Geometry: final body of the model. Coordinates: model frame, mm. A direction names the side the tool comes from. Give positions to 0.01 mm unless a question says otherwise; leave off trailing zeros. Order: outer loops, then holes, each group sorted by start corner. A loop starts at its lowest first (then second) coordinate and runs counter-clockwise, first axis right, second up. Notation, with made-up numbers: (35.25, -31) -> (81.25, -31) arc R14 cw to (81.25, -26) -> close; hole circle Ø11 at (74.25, -35.75). An arc over 180 degrees is marked (long way). One line per question, with ' | ' between items. Start each with the question number.
(1) Mould query, pull axis Y, two halves, no side actions, for faces 1 (the face through (-50, 530, -211)), 2 (the face through (-47, -182, -26)), 3 (the face through (-44.54, 303.72, -67.47)). Classes: +Y half, -Y half, draft (parallel to the pull), parting line (faces both ways), or undercut.
(2) First-contact query: pin 1 Ø8 at (x, z) = (0.5, -979.5) entering from -Y; pin 2 Ø4 at (x, y) = (23, 448.5) entering from -Z; pin 3 Ø5 at (x, y) = (18.5, 178) entering from -Z. Flat tips, straight axial feed; report the tip coordinate or a pass-through.
(3) Ray query, L1, parallel to Y at x = -43, z = -800; L2, parallel to Y at x = -42.55, z = -800; L3, parallel to X at y = 757.5, z = -1069.5. Return the intervals inside material, ascending.
(4) Set-up query: faces 4 (the face through (42, 525, -216)), 5 (the face through (47.54, -533.92, -1382.26)), 6 (the face through (42.76, 474.62, -1418.98)), 7 (the face through (-45, 523, -219)). Return all of +Z, -Z, +X, -X, +Y, -Y with unobstructed straight access to the full face (end or side cutting, diameter ignored); none if empty.
(5) Section A-A (x = -18). Return loops of the section in (y, z), then the cut area to 3 significant figures.
```python
from build123d import *

# Parameters (mm, degrees)
F4_R = 1.5


with BuildPart() as f3:
    # F0 (on Front) → F3 (revolve)
    with BuildSketch(Plane.XZ):
        with BuildLine():
            ThreePointArc((0, 50), (-35.3553390593, 35.3553390593), (-50, 0))
            Line((-50, 0), (-50, -10))
            Line((-50, -10), (-45, -10))
            Line((-45, -10), (-45, -20))
            Line((-45, -20), (-42, -20))
            Line((-42, -20), (-42, -7))
            Line((-42, -7), (-47, -7))
            Line((-47, -7), (-47, 0))
            ThreePointArc((-47, 0), (-33.2340187158, 33.2340187158), (0, 47))
            Line((0, 47), (0, 50))
        make_face()
        with BuildLine():
            ThreePointArc((50, 0), (35.3553390593, 35.3553390593), (0, 50))
            Line((0, 50), (0, 47))
            ThreePointArc((0, 47), (33.2340187158, 33.2340187158), (47, 0))
            Line((47, 0), (47, -7))
            Line((47, -7), (42, -7))
            Line((42, -7), (42, -20))
            Line((42, -20), (45, -20))
            Line((45, -20), (45, -10))
            Line((45, -10), (50, -10))
            Line((50, -10), (50, 0))
        make_face()
    revolve(axis=Axis((11.4029198885, 0, -800), (1, 0, 0)))

    # F4
    f4_edges = [f3.edges().sort_by_distance(p)[0] for p in [
        (45, 0, -1580),
    ]]
    fillet(f4_edges, radius=F4_R)


solid = f3.part
```
Response:
1) face 1: draft | face 2: undercut | face 3: undercut
2) pin 1: stops at y = -831.68 | pin 2: stops at z = -1517.16 | pin 3: stops at z = -1628.62
3) L1: y = -825.51 to -818.97, -793 to -780, 780 to 793, 818.97 to 825.51 | L2: y = -826.26 to -819.96, -793 to -780, 780 to 793, 819.96 to 826.26 | L3: x = -49.84 to -46.83, 46.83 to 49.84
4) face 4: none | face 5: +X | face 6: +X, -X | face 7: -X
5) outline: circle Ø1693.3 at (0, -800); hole circle Ø1686.83 at (0, -800) | area: 17,200 mm^2
